from build123d import *

# Parameters (mm, degrees)
SKETCH1_R           = 7.5
BOSS_EXTRUDE1_DEPTH = 22
SKETCH2_R           = 10
BOSS_EXTRUDE2_DEPTH = 3
SKETCH3_W           = 76.2
SKETCH3_H           = 76.2
BOSS_EXTRUDE3_DEPTH = 10


with BuildPart() as part:
    # Sketch1 → Boss-Extrude1 (new body)
    with BuildSketch(Plane.XY):
        Circle(SKETCH1_R)
    extrude(amount=-BOSS_EXTRUDE1_DEPTH)

    # Sketch2 → Boss-Extrude2 (add)
    with BuildSketch(Plane.XY):
        with Locations(Location((0, 0, 0), (0, 0, 90))):
            Circle(SKETCH2_R)
    extrude(amount=BOSS_EXTRUDE2_DEPTH)

    # Sketch3 → Boss-Extrude3 (add)
    with BuildSketch(Plane.XY.offset(3)):
        Rectangle(SKETCH3_W, SKETCH3_H)
    extrude(amount=BOSS_EXTRUDE3_DEPTH)


solid = part.part
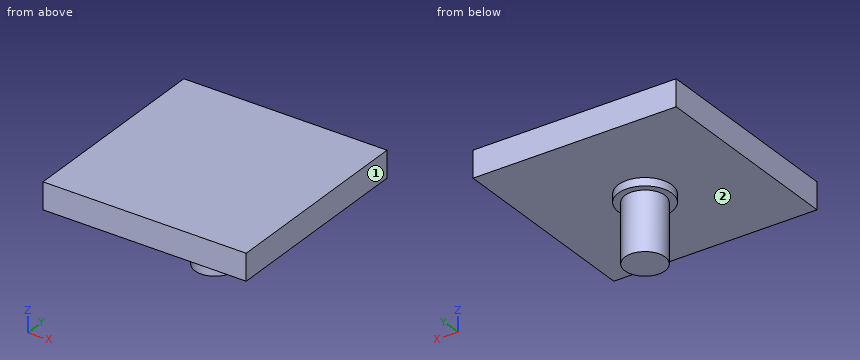
Work out the finished part from the listing and answer in its coordinate system (mm). Face numbers are marked on the shaded views. A direction names the side the tool comes from. Round coordinates to 2 decimals unless told otherwise and drop trailing zeros. Write each loop counter-clockwise with the first axis right and the second up, starting at its lowest first coordinate (ties: lowest second). Pieces come first, ordered by that corner, then holes. Notation, with made-up numbers: M -16.5,53.25 L -8.5,53.25 A20 cw -8.5,86.25 Z; hole C -10,-17.5 d8. An arc over 180 degrees is marked long. Use a Markdown table: item, result.
1) The part is cut by section A-A on y = 0. Give the vertices of the cut face in (x, z), plus the area to 3 significant figures.
Taken from the geometry:
| item | result |
|---|---|
| outline | M -38.1,3 L -10,3 L -10,0 L -7.5,0 L -7.5,-22 L 7.5,-22 L 7.5,0 L 10,0 L 10,3 L 38.1,3 L 38.1,13 L -38.1,13 Z |
| area | 1,150 mm2 |
2) The part is cut by section C-C on z = -3. Give the vertices of the cut face in (x, y), plus the area to 3 significant figures.
Taken from the geometry:
| item | result |
|---|---|
| outline | C 0,0 d15 |
| area | 177 mm2 |
3) Consider line 1 (Z direction, x = -18.5, y = 24); line 2 (X direction, y = -1, z = -14); line 3 (X direction, y = -5.5, z = -1.5). Determine where each line is inside the solid, lowest interval first. Write a range as [from, to].
Taken from the geometry:
| item | result |
|---|---|
| line 1 | z = [3, 13] |
| line 2 | x = [-7.43, 7.43] |
| line 3 | x = [-5.1, 5.1] |
4) The part is cut by section D-D on x = 32. Give the vertices of the cut face in (y, z).
Taken from the geometry:
| item | result |
|---|---|
| outline | M -38.1,3 L 38.1,3 L 38.1,13 L -38.1,13 Z |
5) Which of the six approach directions +Z, -Z, +X, -X, +Y, -Y give full straight-line access (tool end or side, diameter ignored) to the marked faces 1 and 2?
Taken from the geometry:
| item | result |
|---|---|
| face 1 | +Z, -Z, +X, +Y, -Y |
| face 2 | -Z |
6) Flat-ended cylindrical pins translate along their axes: pin 1 (2 mm diameter, centred on x = -11.5, y = -24, fed in from -Z); pin 2 (6 mm diameter, centred on x = 0, z = -7.5, fed in from +Y). Find the tip coordinate at first contact, or state that the pin passes through.
Taken from the geometry:
| item | result |
|---|---|
| pin 1 | stops at z = 3 |
| pin 2 | stops at y = 7.5 |
